from build123d import *

# Parameters (mm, degrees)
SKETCH_1_R      = 31
SKETCH_1_R_2    = 1.6
SKETCH_1_R_3    = 21.1
EXTRUDE_1_DEPTH = 15
EXTRUDE_START   = -10
SKETCH_2_R      = 21.1
SKETCH_2_R_2    = 13.2
SKETCH_2_R_3    = 2.2
EXTRUDE_2_DEPTH = 5


with BuildPart() as part:
    # 草图1 → 凸台-拉伸1 (new body)
    # profile 1 of 3: a face of its own
    with BuildSketch(Plane(origin=(0, 0, 0), x_dir=(1, 0, 0), z_dir=(0, 1, 0))):
        Circle(SKETCH_1_R)
        with Locations(Location((-18.384776311, 18.384776311, 0), (0, 0, 270))):
            Circle(SKETCH_1_R_2, mode=Mode.SUBTRACT)
        with Locations(Location((-18.384776311, -18.384776311, 0), (0, 0, 270))):
            Circle(SKETCH_1_R_2, mode=Mode.SUBTRACT)
        with Locations(Location((18.384776311, -18.384776311, 0), (0, 0, 270))):
            Circle(SKETCH_1_R_2, mode=Mode.SUBTRACT)
        with Locations(Location((18.384776311, 18.384776311, 0), (0, 0, 270))):
            Circle(SKETCH_1_R_2, mode=Mode.SUBTRACT)
        with Locations(Location((0, 0, 0), (0, 0, 270))):
            Circle(SKETCH_1_R_3, mode=Mode.SUBTRACT)
    # profile 2 of 3: a face of its own
    with BuildSketch(Plane(origin=(0, 0, 0), x_dir=(1, 0, 0), z_dir=(0, 1, 0))):
        with BuildLine():
            Line((-31, 31), (-31, 0))
            ThreePointArc((-31, 0), (-21.920310218, 21.920310215), (-4e-09, 31))
            Line((-4e-09, 31), (-31, 31))
        make_face()
    # profile 3 of 3: a face of its own
    with BuildSketch(Plane(origin=(0, 0, 0), x_dir=(1, 0, 0), z_dir=(0, 1, 0))):
        with BuildLine():
            ThreePointArc((-4e-09, 31), (21.920310215, 21.920310218), (31, 0))
            Line((31, 0), (31, 31))
            Line((31, 31), (-4e-09, 31))
        make_face()
    extrude(amount=EXTRUDE_1_DEPTH)

    # 草图2 → 凸台-拉伸2 (add)
    with BuildSketch(Plane.XZ.offset(EXTRUDE_START)):
        with Locations(Location((0, 0, 0), (0, 0, 270))):
            Circle(SKETCH_2_R)
        with Locations(Location((0, 0, 0), (0, 0, 270))):
            Circle(SKETCH_2_R_2, mode=Mode.SUBTRACT)
        with Locations(Location((0, 17.5, 0), (0, 0, 270))):
            Circle(SKETCH_2_R_3, mode=Mode.SUBTRACT)
        with Locations(Location((17.5, 0, 0), (0, 0, 270))):
            Circle(SKETCH_2_R_3, mode=Mode.SUBTRACT)
        with Locations(Location((0, -17.5, 0), (0, 0, 270))):
            Circle(SKETCH_2_R_3, mode=Mode.SUBTRACT)
        with Locations(Location((-17.5, 0, 0), (0, 0, 270))):
            Circle(SKETCH_2_R_3, mode=Mode.SUBTRACT)
    extrude(amount=-EXTRUDE_2_DEPTH)


solid = part.part
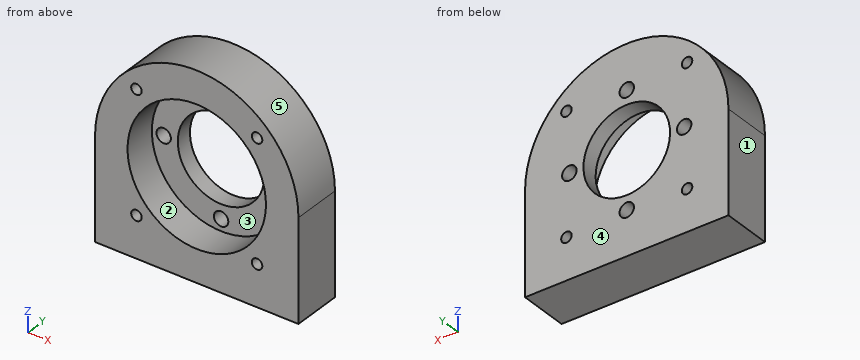
Part model, mm, in its own coordinate system. Face numbers are marked on the shaded views. A direction names the side the tool comes from. Give positions to 0.01 mm unless a question says otherwise; leave off trailing zeros. Order: outer loops, then holes, each group sorted by start corner. A loop starts at its lowest first (then second) coordinate and runs counter-clockwise, first axis right, second up. Notation, with made-up numbers: (21.5, 14) - (27.5, 14) arc R29 cw to (27.5, 40) - close; hole circle Ø8 at (89.25, 73). An arc over 180 degrees is marked (long way). One line per question, with ' | ' between items.
1. Band-saw the part on A-A on x = 0. List the corners of the cut face in (y, z).
Filled in:
outline: (0, -31) - (15, -31) - (15, -19.7) - (10, -19.7) - (10, -21.1) - (0, -21.1) - close; (0, 21.1) - (10, 21.1) - (10, 19.7) - (15, 19.7) - (15, 31) - (0, 31) - close; (10, -15.3) - (15, -15.3) - (15, -13.2) - (10, -13.2) - close; (10, 13.2) - (15, 13.2) - (15, 15.3) - (10, 15.3) - close
2. Drill centre lines: probe 1 along X at (y, z) = (13.7, 0); probe 2 along Z at (x, y) = (-19, 7.5); probe 3 along X at (y, z) = (6.75, -17). Where is each one in solid material? Low to high.
Filled in:
probe 1: -31 to -19.7, -15.3 to -13.2, 13.2 to 15.3, 19.7 to 31 | probe 2: -31 to -19.86, -16.91 to -9.18, 9.18 to 16.91, 19.86 to 24.49 | probe 3: -31 to -19.19, -17.58 to -12.5, 12.5 to 17.58, 19.19 to 31
3. Band-saw the part on B-B on z = -7. List the corners of the cut face in (x, y).
Filled in:
outline: (-31, 0) - (-19.91, 0) - (-19.91, 10) - (-11.19, 10) - (-11.19, 15) - (-31, 15) - close; (11.19, 10) - (19.91, 10) - (19.91, 0) - (31, 0) - (31, 15) - (11.19, 15) - close
4. Pull direction Z, two halves, no side cores. Call the marked faces 3, 4 and 5: +Z half, -Z half, draft (parallel to the pull), parting line (faces both ways), or undercut.
Filled in:
face 3: undercut | face 4: draft | face 5: +Z half
5. Drop flat-ended pins along their axis: P1, Ø4, axis at x = 0, z = 17.5, coming from the +Y side; P2, Ø8, axis at x = -9.5, y = 9, coming from the +Z side; P3, Ø8, axis at x = -5.5, y = 2.5, coming from the +Z side; P4, Ø3, axis at y = 6, z = 14.5, coming from the +X side. Give the stop position or say it passes through.
Filled in:
P1: through | P2: z = 30.51 | P3: z = 30.96 | P4: x = 28.14
6. Which spindle directions (+Z, -Z, +X, -X, +Y, -Y) get a long thin tool onto all of the face, cutting with end or side? Do the marked faces 1 and 2. Say none if no direction does.
Filled in:
face 1: +Z, -Z, -X, +Y, -Y | face 2: -Y
7. Band-saw the part on C-C on y = 5. List the corners of the cut face in (x, z).
Filled in:
outline: (-31, -31) - (31, -31) - (31, 0) arc R31 ccw to (-31, 0) - close; hole circle Ø42.2 at (0, 0); hole circle Ø3.2 at (-18.38, -18.38); hole circle Ø3.2 at (-18.38, 18.38); hole circle Ø3.2 at (18.38, -18.38); hole circle Ø3.2 at (18.38, 18.38)
8. Band-saw the part on D-D on x = -7.5. List the corners of the cut face in (y, z), then the cut area to 3 significant figures.
Filled in:
outline: (0, -31) - (15, -31) - (15, -10.86) - (10, -10.86) - (10, -19.72) - (0, -19.72) - close; (0, 19.72) - (10, 19.72) - (10, 10.86) - (15, 10.86) - (15, 30.08) - (0, 30.08) - close | area: 413 mm²
